from build123d import *

# Parameters (mm, degrees)
CROQUIS1_R              = 70
CROQUIS1_R_2            = 4.5
CROQUIS1_R_3            = 3.25
SALIENTE_EXTRUIR1_DEPTH = 3


with BuildPart() as part:
    # Croquis1 → Saliente-Extruir1 (new body)
    with BuildSketch(Plane(origin=(0, 0, 0), x_dir=(1, 0, 0), z_dir=(0, 1, 0))):
        with Locations(Location((0, 0, 0), (0, 0, 270))):
            Circle(CROQUIS1_R)
        with Locations(Location((0, 0, 0), (0, 0, 270))):
            Circle(CROQUIS1_R_2, mode=Mode.SUBTRACT)
        with Locations(Location((0, -50, 0), (0, 0, 270))):
            Circle(CROQUIS1_R_3, mode=Mode.SUBTRACT)
        Polygon((24.748737342, 24.748737342), (29.69848481, 19.798989873), (31.819805153, 21.920310217), (21.920310217, 31.819805153), (19.798989873, 29.69848481), align=None, mode=Mode.SUBTRACT)
        Polygon((24.748737342, -24.748737342), (19.798989873, -29.69848481), (21.920310217, -31.819805153), (31.819805153, -21.920310217), (29.69848481, -19.798989873), align=None, mode=Mode.SUBTRACT)
        Polygon((-24.748737342, 24.748737342), (-19.798989873, 29.69848481), (-21.920310217, 31.819805153), (-31.819805153, 21.920310217), (-29.69848481, 19.798989873), align=None, mode=Mode.SUBTRACT)
        Polygon((-24.748737342, -24.748737342), (-29.69848481, -19.798989873), (-31.819805153, -21.920310217), (-21.920310217, -31.819805153), (-19.798989873, -29.69848481), align=None, mode=Mode.SUBTRACT)
        Polygon((0, 62), (20, 62), (20, 59), (-20, 59), (-20, 62), align=None, mode=Mode.SUBTRACT)
        Polygon((55.861435714, 27.577164466), (27.577164466, 55.861435714), (29.69848481, 57.982756057), (43.840620434, 43.840620434), (57.982756057, 29.69848481), align=None, mode=Mode.SUBTRACT)
        Polygon((59, -20), (59, 20), (62, 20), (62, 0), (62, -20), align=None, mode=Mode.SUBTRACT)
        Polygon((27.577164466, -55.861435714), (55.861435714, -27.577164466), (57.982756057, -29.69848481), (43.840620434, -43.840620434), (29.69848481, -57.982756057), align=None, mode=Mode.SUBTRACT)
        Polygon((-20, -59), (20, -59), (20, -62), (0, -62), (-20, -62), align=None, mode=Mode.SUBTRACT)
        Polygon((-55.861435714, -27.577164466), (-27.577164466, -55.861435714), (-29.69848481, -57.982756057), (-43.840620434, -43.840620434), (-57.982756057, -29.69848481), align=None, mode=Mode.SUBTRACT)
        Polygon((-59, 20), (-59, -20), (-62, -20), (-62, 0), (-62, 20), align=None, mode=Mode.SUBTRACT)
        Polygon((-27.577164466, 55.861435714), (-55.861435714, 27.577164466), (-57.982756057, 29.69848481), (-43.840620434, 43.840620434), (-29.69848481, 57.982756057), align=None, mode=Mode.SUBTRACT)
    extrude(amount=SALIENTE_EXTRUIR1_DEPTH)


solid = part.part
Work out the finished part from the listing and answer in its coordinate system (mm). Give positions to 0.01 mm unless a question says otherwise; leave off trailing zeros. Write each loop counter-clockwise with the first axis right and the second up, starting at its lowest first coordinate (ties: lowest second). Pieces come first, ordered by that corner, then holes.
Q1. Given pin 1 (1.5 mm diameter, centred on y = 1.5, z = -5, fed in from +X); pin 2 (1.5 mm diameter, centred on x = -60.5, y = 1, fed in from +Z); pin 3 (1.5 mm diameter, centred on y = 2, z = 61, fed in from -X), each flat-ended and moving along its own axis, determine where each tip first touches the part or whether it passes through.
Answer:
pin 1: stops at x = 69.87
pin 2: stops at z = 36.47
pin 3: stops at x = -35.64
Q2. The part is cut by section B-B on x = -33.5. Give the vertices of the cut face in (y, z), and give its area (3 significant figures).
Answer:
outline: (0, -61.46) - (3, -61.46) - (3, -54.18) - (0, -54.18) - close; (0, -49.94) - (3, -49.94) - (3, 49.94) - (0, 49.94) - close; (0, 54.18) - (3, 54.18) - (3, 61.46) - (0, 61.46) - close
area: 343 mm2
Q3. For a pull along X with two mould halves and no side action, classify faces 1 (the face through (-42.594, 1.479, -55.55)), 2 (the face through (61, 1, 20)), 3 (the face through (1, 0, -17)) as released by +X, released by -X, zero draft, split by the parting line, or undercut.
Answer:
face 1: split by the parting line
face 2: undercut
face 3: zero draft
Q4. The part is cut by section D-D on y = 1.7. State how many separate pieces and enclosed holes the cut face has, and give its area (3 significant figures).
Answer:
separate pieces: 1
enclosed holes: 14
area: 14,200 mm2
Q5. The part is cut by section A-A on z = 0. Give the vertices of the cut face in (x, y).
Answer:
outline: (-70, 0) - (-62, 0) - (-62, 3) - (-70, 3) - close; (-59, 0) - (-4.5, 0) - (-4.5, 3) - (-59, 3) - close; (4.5, 0) - (59, 0) - (59, 3) - (4.5, 3) - close; (62, 0) - (70, 0) - (70, 3) - (62, 3) - close
Q6. The part is cut by section C-C on z = -42. Give the vertices of the cut face in (x, y).
Answer:
outline: (-56, 0) - (-45.68, 0) - (-45.68, 3) - (-56, 3) - close; (-41.44, 0) - (41.44, 0) - (41.44, 3) - (-41.44, 3) - close; (45.68, 0) - (56, 0) - (56, 3) - (45.68, 3) - close
Q7. Straight lines are drawn through the part: L1, parallel to X at y = 1.05, z = 0; L2, parallel to X at y = 2.1, z = 11; L3, parallel to X at y = 1, z = 50. For each, find the intervals that lie inside material, in ascending order.
Answer:
L1: x = -70 to -62, -59 to -4.5, 4.5 to 59, 62 to 70
L2: x = -69.13 to -62, -59 to 59, 62 to 69.13
L3: x = -48.99 to -37.68, -33.44 to -3.25, 3.25 to 33.44, 37.68 to 48.99
